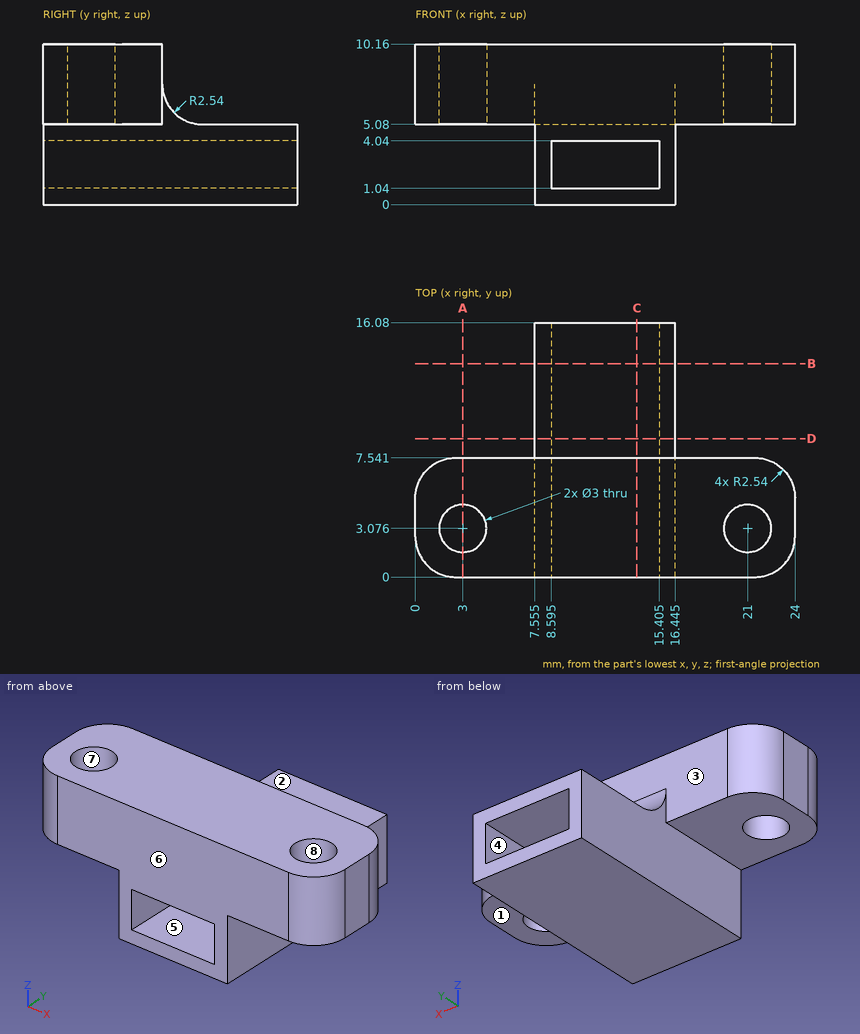
Geometry: see drawing. Coordinates: mm, zero at the bounding-box minimum. A direction names the side the tool comes from. Coordinates: 2 decimals unless noted, no trailing zeros. Order: outer loops, then holes, each group sorted by start corner. A loop starts at its lowest first (then second) coordinate and runs counter-clockwise, first axis right, second up. Notation, with made-up numbers: (38.25, 28.5) - (78.25, 28.5) arc R25 ccw to (78.25, 47.5) - close; hole circle Ø5 at (67, -23). An arc over 180 degrees is marked (long way). Write each question's results on one line, items separated by ' | '.
1) Set-up query: the marked faces 1, 2, 3 and 4. Return all of +Z, -Z, +X, -X, +Y, -Y with unobstructed straight access to the full face (end or side cutting, diameter ignored); none if empty.
Results list:
face 1: -Z, +X, +Y, -Y | face 2: +Z, +X, -X, +Y | face 3: +Z, +Y | face 4: +Y, -Y
2) Section C-C, the plane x = 14. Return loops of the section in (y, z).
Results list:
outline: (0, 0) - (16.08, 0) - (16.08, 1.04) - (0, 1.04) - close; (0, 4.04) - (16.08, 4.04) - (16.08, 5.08) - (10.08, 5.08) arc R2.54 cw to (7.54, 7.62) - (7.54, 10.16) - (0, 10.16) - close
3) Pin query (flat end, axial travel): pin 1 (2.5 mm diameter, centred on y = 4.5, z = 3.5, fed in from +X) (1 decimal); pin 2 (2.5 mm diameter, centred on y = 10, z = 3, fed in from -X) (1 decimal); pin 3 (3 mm diameter, centred on x = 14, y = 13.5, fed in from +Z). Return the tip coordinate at first contact, or that it passes through.
Results list:
pin 1: x = 16.4 | pin 2: x = 7.6 | pin 3: z = 5.08
4) Line query: line 1 (Z direction, x = 14.5, y = 14.25); line 2 (Y direction, x = 21, z = 6.75) (1 decimal); line 3 (X direction, y = 10.25, z = 3.5) (1 decimal). Output: solid intervals per line, ascending. Write a range as from..to.
Results list:
line 1: 0..1.04, 4.04..5.08 | line 2: 0..1.6, 4.6..7.5 | line 3: 7.6..8.6, 15.4..16.4
5) Section A-A, the plane x = 3. Return loops of the section in (y, z) (1 decimal).
Results list:
outline: (0, 5.1) - (1.6, 5.1) - (1.6, 10.2) - (0, 10.2) - close; (4.6, 5.1) - (7.5, 5.1) - (7.5, 10.2) - (4.6, 10.2) - close
6) Pull-direction query (Y, two-part tool) for the marked faces 5, 6, 7 and 8; classes: pulls with the +Y half, pulls with the -Y half, needs draft (parallel to the pull), parting line crosses it, or undercut.
Results list:
face 5: needs draft | face 6: pulls with the -Y half | face 7: undercut | face 8: undercut
7) Section B-B, the plane y = 13.5. Return loops of the section in (x, z) (1 decimal).
Results list:
outline: (7.6, 0) - (16.4, 0) - (16.4, 5.1) - (7.6, 5.1) - close; hole (8.6, 1) - (15.4, 1) - (15.4, 4) - (8.6, 4) - close
8) Section D-D, the plane y = 8.75. Return loops of the section in (x, z) (1 decimal).
Results list:
outline: (7.6, 0) - (16.4, 0) - (16.4, 5.5) - (7.6, 5.5) - close; hole (8.6, 1) - (15.4, 1) - (15.4, 4) - (8.6, 4) - close
